Could you check a few things on this drawing? It's one solid part, dimensions in mm from its lowest x, y, z. A direction names the side the tool comes from. Coordinates: 2 decimals unless noted, no trailing zeros. Write each loop counter-clockwise with the first axis right and the second up, starting at its lowest first coordinate (ties: lowest second). Pieces come first, ordered by that corner, then holes. Notation, with made-up numbers: (84, -11) - (108, -11) arc R26 ccw to (108, 24) - close; hole circle Ø8 at (74.5, 52). An arc over 180 degrees is marked (long way). Write item = value, one per line. Start each with the question number.
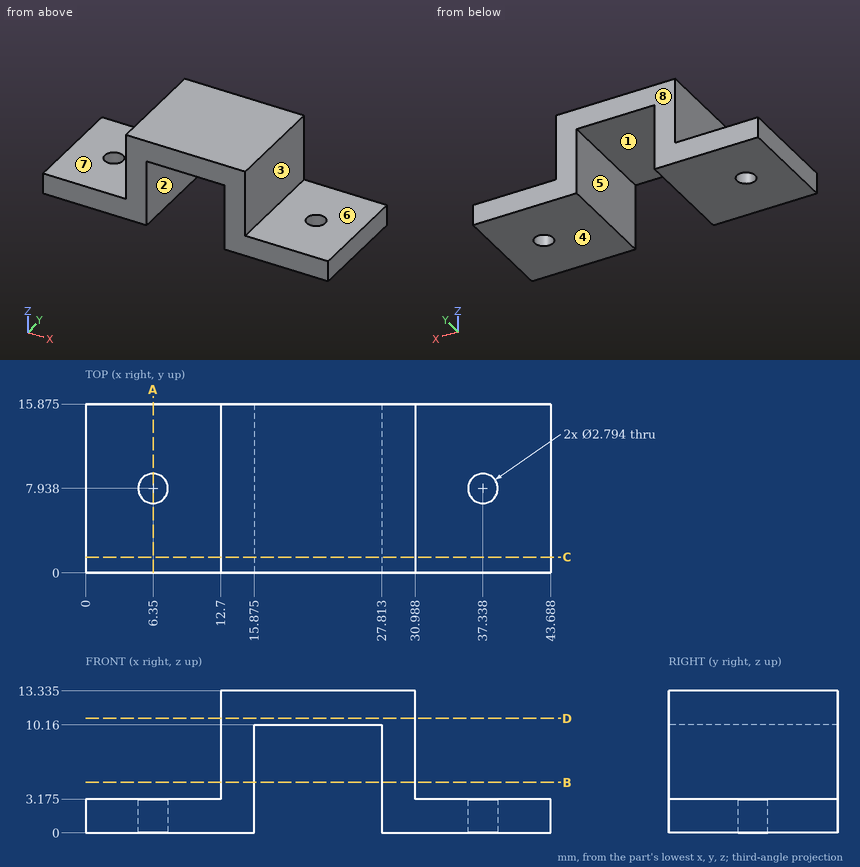
1) Suppose I cut it at A-A on x = 6.35. Please give me the cut outline in (y, z) (1 decimal).
2) Suppose I cut it at C-C on y = 1.5. Please give me the cut outline in (x, z) (1 decimal).
3) If I drill on probe 1 along X at (y, z) = (3.25, 1.75) (1 decimal); probe 2 along Y at (x, z) = (6.35, 2.05) (1 decimal); probe 3 along X at (y, z) = (3, 6.75) (1 decimal), over which ranges is the centre line in solid material (lowest first)? Write a range as [from, to].
4) Thinking about a two-plate mould opening in X: for the marked faces 1, 2, 3 and 4, which applies, +X half, -X half, draft (parallel to the pull), parting line (faces both ways), or undercut?
5) Suppose I cut it at D-D on z = 10.75. Please give me the cut outline in (x, y) (1 decimal), plus the area to 3 significant figures.
6) Suppose I cut it at B-B on z = 4.75. Please give me the cut outline in (x, y) (1 decimal).
7) For P1, Ø8, axis at y = 5.5, z = 12, coming from the -X side; P2, Ø8, axis at x = 11, y = 9, coming from the -Z side; P3, Ø5, axis at y = 7, z = 7.5, coming from the +X side; P4, Ø2, axis at x = 6.35, y = 7.94, coming from the -Z side, each with a flat end and sliding along its axis, tell me the tip position at first contact or that it passes through.
8) Which directions (+Z, -Z, +X, -X, +Y, -Y) give clear straight access to the entire face, cutting with the end or side of a thin tool? Please do the marked faces 5, 6, 7 and 8.
Reply:
q1.outline = (0, 0) - (6.5, 0) - (6.5, 3.2) - (0, 3.2) - close; (9.3, 0) - (15.9, 0) - (15.9, 3.2) - (9.3, 3.2) - close
q2.outline = (0, 0) - (15.9, 0) - (15.9, 10.2) - (27.8, 10.2) - (27.8, 0) - (43.7, 0) - (43.7, 3.2) - (31, 3.2) - (31, 13.3) - (12.7, 13.3) - (12.7, 3.2) - (0, 3.2) - close
q3.probe_1 = [0, 15.9], [27.8, 43.7]
q3.probe_2 = [0, 6.5], [9.3, 15.9]
q3.probe_3 = [12.7, 15.9], [27.8, 31]
q4.face_1 = undercut
q4.face_2 = undercut
q4.face_3 = +X half
q4.face_4 = draft
q5.outline = (12.7, 0) - (31, 0) - (31, 15.9) - (12.7, 15.9) - close
q5.area = 290 mm^2
q6.outline = (12.7, 0) - (15.9, 0) - (15.9, 15.9) - (12.7, 15.9) - close; (27.8, 0) - (31, 0) - (31, 15.9) - (27.8, 15.9) - close
q7.P1 = 12.7
q7.P2 = 0
q7.P3 = 30.99
q7.P4 = through
q8.face_5 = -Z, +Y, -Y
q8.face_6 = +Z, +X, +Y, -Y
q8.face_7 = +Z, -X, +Y, -Y
q8.face_8 = +Z, -Z, +X, -X, +Y
